Check sheet for the modelled part. Datum: model origin and axes. Units: mm. A direction names the side the tool comes from. Give positions to 0.01 mm unless a question says otherwise; leave off trailing zeros. Order: outer loops, then holes, each group sorted by start corner. A loop starts at its lowest first (then second) coordinate and runs counter-clockwise, first axis right, second up.
from build123d import *

# Parameters (mm, degrees)
CYLINDER005_R               = 2.5
CYLINDER005_DEPTH           = 27
CYLINDER005_PLACEMENT_ANGLE = 89.999981
CYLINDER004_R               = 2.5
CYLINDER004_DEPTH           = 27
CYLINDER004_PLACEMENT_ANGLE = 89.999981
BOX004_W                    = 6.5
BOX004_H                    = 9
BOX004_DEPTH                = 18
BOX003_W                    = 24
BOX003_H                    = 7
BOX003_DEPTH                = 34
BOX005_W                    = 6.5
BOX005_H                    = 9
BOX005_DEPTH                = 18
BOX_W                       = 42
BOX_H                       = 22
BOX_DEPTH                   = 18
CYLINDER001_R               = 2.75
CYLINDER001_DEPTH           = 18
CYLINDER002_R               = 2.75
CYLINDER002_DEPTH           = 18
CYLINDER003_R               = 2.75
CYLINDER003_DEPTH           = 18
CYLINDER_R                  = 2.75
CYLINDER_DEPTH              = 18
BOX002_W                    = 58
BOX002_H                    = 35
BOX002_DEPTH                = 7.5


with BuildPart() as cylinder005:
    # Cylinder005 → Cylinder005 (new body)
    with BuildSketch(Plane.XY):
        Circle(CYLINDER005_R)
    extrude(amount=CYLINDER005_DEPTH)


with BuildPart() as cylinder005_1:
    # Cylinder005 placement: moved
    add(cylinder005.part.moved(Location((-2, -19.5, -10))).rotate(Axis((-2, -19.5, -10), (0, 1, 0)), CYLINDER005_PLACEMENT_ANGLE))


with BuildPart() as fusion003:
    # Cylinder004 → Cylinder004 (new body)
    with BuildSketch(Plane.XY):
        Circle(CYLINDER004_R)
    extrude(amount=CYLINDER004_DEPTH)


with BuildPart() as fusion003_1:
    # Cylinder004 placement: moved
    add(fusion003.part.moved(Location((-2, -19.5, -19))).rotate(Axis((-2, -19.5, -19), (0, 1, 0)), CYLINDER004_PLACEMENT_ANGLE))

    # Fusion003: union Cylinder005
    add(cylinder005_1.part)


with BuildPart() as cube001:
    # Box004 → Box004 (new body)
    with BuildSketch(Plane(origin=(-0.5, -24, -23.5), x_dir=(1, 0, 0), z_dir=(0, 0, 1))):
        with Locations((3.25, 4.5)):
            Rectangle(BOX004_W, BOX004_H)
    extrude(amount=BOX004_DEPTH)


with BuildPart() as cube:
    # Box003 → Box003 (new body)
    with BuildSketch(Plane(origin=(-0.5, -15, -23.5), x_dir=(1, 0, 0), z_dir=(0, 0, 1))):
        with Locations((12, 3.5)):
            Rectangle(BOX003_W, BOX003_H)
    extrude(amount=BOX003_DEPTH)


with BuildPart() as module_hole_der:
    # Box005 → Box005 (new body)
    with BuildSketch(Plane(origin=(17, -24, -23.5), x_dir=(1, 0, 0), z_dir=(0, 0, 1))):
        with Locations((3.25, 4.5)):
            Rectangle(BOX005_W, BOX005_H)
    extrude(amount=BOX005_DEPTH)

    # Fusion002: union Cube001, Cube
    add(cube001.part)
    add(cube.part)

    # Cut001: cut Fusion003
    add(fusion003_1.part, mode=Mode.SUBTRACT)


with BuildPart() as servo_mold:
    # Box → Box (new body)
    with BuildSketch(Plane(origin=(-1, -1, 0), x_dir=(1, 0, 0), z_dir=(0, 0, 1))):
        with Locations((21, 11)):
            Rectangle(BOX_W, BOX_H)
    extrude(amount=BOX_DEPTH)


with BuildPart() as hole002:
    # Cylinder001 → Cylinder001 (new body)
    with BuildSketch(Plane(origin=(-4.5, 15.5, 0), x_dir=(1, 0, 0), z_dir=(0, 0, 1))):
        Circle(CYLINDER001_R)
    extrude(amount=CYLINDER001_DEPTH)


with BuildPart() as hole003:
    # Cylinder002 → Cylinder002 (new body)
    with BuildSketch(Plane(origin=(44.5, 4.5, 0), x_dir=(1, 0, 0), z_dir=(0, 0, 1))):
        Circle(CYLINDER002_R)
    extrude(amount=CYLINDER002_DEPTH)


with BuildPart() as hole004:
    # Cylinder003 → Cylinder003 (new body)
    with BuildSketch(Plane(origin=(44.5, 15.5, 0), x_dir=(1, 0, 0), z_dir=(0, 0, 1))):
        Circle(CYLINDER003_R)
    extrude(amount=CYLINDER003_DEPTH)


with BuildPart() as servo_object:
    # Cylinder → Cylinder (new body)
    with BuildSketch(Plane(origin=(-4.5, 4.5, 0), x_dir=(1, 0, 0), z_dir=(0, 0, 1))):
        Circle(CYLINDER_R)
    extrude(amount=CYLINDER_DEPTH)

    # Fusion: union Hole002, Hole003, Hole004
    add(hole002.part)
    add(hole003.part)
    add(hole004.part)

    # Fusion001: union Servo Mold
    add(servo_mold.part)


with BuildPart() as complete_arm_holder:
    # Box002 → Box002 (new body)
    with BuildSketch(Plane(origin=(-9, -15, 10.5), x_dir=(1, 0, 0), z_dir=(0, 0, 1))):
        with Locations((29, 17.5)):
            Rectangle(BOX002_W, BOX002_H)
    extrude(amount=BOX002_DEPTH)

    # Cut: cut Servo Object
    add(servo_object.part, mode=Mode.SUBTRACT)

    # Fusion004: union Module Hole-der
    add(module_hole_der.part)


solid = complete_arm_holder.part
1) Depth check by flat-ended pin: pin 1 Ø3 at (x, z) = (-1, 3) entering from +Y; pin 2 Ø3 at (x, y) = (4, -21) entering from +Z; pin 3 Ø8 at (y, z) = (-14, 0) entering from -X. Enter the tip coordinate at first touch or a pass-through.
Recorded:
pin 1: stops at y = -8
pin 2: stops at z = -5.5
pin 3: stops at x = -0.5
2) Set-up check for faces 1 (the face through (-1, 9, 14)), 2 (the face through (-0.5, -14, -11)), 3 (the face through (2.7, -17.39, -11.34)), 4 (the face through (3, -19, -5.5)), 5 (the face through (17, -20, -15)): record each of +Z, -Z, +X, -X, +Y, -Y from which the full face is reachable in a straight line by a thin tool's end or side.
Recorded:
face 1: +Z, -Z, +Y
face 2: -Z, -X, +Y, -Y
face 3: +X, -X
face 4: +Z, +X, -X, -Y
face 5: +Z, -Z, -Y
3) Section check C-C, the plane y = 4.5. Record the cut outline in (x, z), then the cut area to 3 significant figures.
Recorded:
outline: (-9, 10.5) - (-7.25, 10.5) - (-7.25, 18) - (-9, 18) - close; (-1.75, 10.5) - (-1, 10.5) - (-1, 18) - (-1.75, 18) - close; (41, 10.5) - (41.75, 10.5) - (41.75, 18) - (41, 18) - close; (47.25, 10.5) - (49, 10.5) - (49, 18) - (47.25, 18) - close
area: 37.5 mm2
4) Section check D-D, the plane z = -19. State how many separate pieces and enclosed holes the cut face has, then the cut area to 3 significant figures.
Recorded:
separate pieces: 3
enclosed holes: 0
area: 220 mm2
5) Draft check along X on faces 6 (the face through (-3.23, 2.06, 14.2)), 7 (the face through (49, 2, 14)), 8 (the face through (-9, 2, 14)). Enter one of: +X half, -X half, draft (parallel to the pull), parting line (faces both ways), or undercut.
Recorded:
face 6: undercut
face 7: +X half
face 8: -X half
6) Section check A-A, the plane x = 44.5. Record the cut outline in (y, z).
Recorded:
outline: (-15, 10.5) - (1.75, 10.5) - (1.75, 18) - (-15, 18) - close; (7.25, 10.5) - (12.75, 10.5) - (12.75, 18) - (7.25, 18) - close; (18.25, 10.5) - (20, 10.5) - (20, 18) - (18.25, 18) - close
7) Material ranges on L1, parallel to Z at x = 2, y = -19.5; L2, parallel to X at y = 15.5, z = 13.75; L3, parallel to Y at x = -4.5, z = 13, recorded low to high.
Recorded:
L1: z = -23.5 to -21.5, -16.5 to -12.5, -7.5 to -5.5
L2: x = -9 to -7.25, -1.75 to -1, 41 to 41.75, 47.25 to 49
L3: y = -15 to 1.75, 7.25 to 12.75, 18.25 to 20
8) Section check B-B, the plane y = -19.5. Record the cut outline in (x, z).
Recorded:
outline: (-0.5, -23.5) - (6, -23.5) - (6, -21.5) - (-0.5, -21.5) - close; (-0.5, -16.5) - (6, -16.5) - (6, -12.5) - (-0.5, -12.5) - close; (-0.5, -7.5) - (6, -7.5) - (6, -5.5) - (-0.5, -5.5) - close; (17, -23.5) - (23.5, -23.5) - (23.5, -21.5) - (17, -21.5) - close; (17, -16.5) - (23.5, -16.5) - (23.5, -12.5) - (17, -12.5) - close; (17, -7.5) - (23.5, -7.5) - (23.5, -5.5) - (17, -5.5) - close
